from build123d import *

# Parameters (mm, degrees)
EXTRUDE_1_DEPTH     = 455
SKETCH_3_R          = 2.1
CUT_EXTRUDE_1_DEPTH = 466.453246739
SKETCH_7_W          = 87.07
SKETCH_7_H          = 105
CUT_EXTRUDE_2_DEPTH = 10


with BuildPart() as part:
    # 草图2 → 凸台-拉伸1 (new body)
    with BuildSketch(Plane.XY):
        Polygon((-98, -1), (-96.845299462, 1), (96.915299462, 1), (98.07, -1), align=None)
    extrude(amount=-EXTRUDE_1_DEPTH)

    # 草图3 → 切除-拉伸1 (cut, through all)
    with BuildSketch(Plane(origin=(0, -1, 0), x_dir=(-1, 0, 0), z_dir=(0, -1, 0))):
        with Locations(Location((78, 35, 0), (0, 0, 90))):
            Circle(SKETCH_3_R)
        with Locations(Location((78, 55, 0), (0, 0, 90))):
            Circle(SKETCH_3_R)
        with Locations(Location((-78, 55, 0), (0, 0, 270))):
            Circle(SKETCH_3_R)
        with Locations(Location((-78, 35, 0), (0, 0, 270))):
            Circle(SKETCH_3_R)
        with Locations(Location((-78, 420, 0), (0, 0, 90))):
            Circle(SKETCH_3_R)
        with Locations(Location((-78, 400, 0), (0, 0, 90))):
            Circle(SKETCH_3_R)
        with Locations(Location((78, 400, 0), (0, 0, 270))):
            Circle(SKETCH_3_R)
        with Locations(Location((78, 420, 0), (0, 0, 270))):
            Circle(SKETCH_3_R)
    extrude(amount=-CUT_EXTRUDE_1_DEPTH, mode=Mode.SUBTRACT)

    # 草图7 → 切除-拉伸2 (cut)
    with BuildSketch(Plane.XZ.offset(1)):
        with Locations((0.035, -302.5)):
            Rectangle(SKETCH_7_W, SKETCH_7_H)
    extrude(amount=-CUT_EXTRUDE_2_DEPTH, mode=Mode.SUBTRACT)


solid = part.part
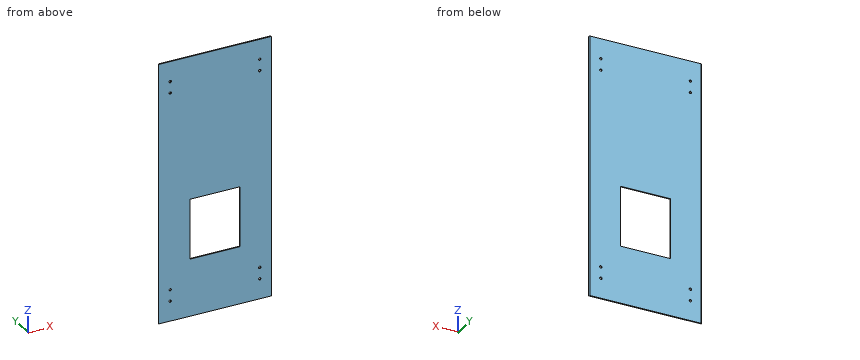
Input: part model. Units: mm. Frame: model coordinates. Give positions to 0.01 mm unless a question says otherwise; leave off trailing zeros. Write each loop counter-clockwise with the first axis right and the second up, starting at its lowest first coordinate (ties: lowest second). Pieces come first, ordered by that corner, then holes. Notation, with made-up numbers: M 46.5,78.25 L 72.5,78.25 A11 ccw 72.5,90.25 Z; hole C -13,76.25 d10. An arc over 180 degrees is marked long. Write item = value, one per line. Start each with the question number.
1) Cut plane B-B on z = -298.5. Return the cut outline in (x, y).
2) Material intervals for line 1 along X through (y, z) = (-0.5, -400); line 2 along Z through (x, y) = (-5.5, 0.65); line 3 along X through (y, z) = (0.8, -55), sorted ascending. Write a range as [from, to].
3) Cut plane C-C on y = -0.65. Count the separate pieces of the cut face and the enclosed holes in it, then the cut area to 3 significant figures.
4) First-contact query: pin 1 Ø1 at (y, z) = (0.5, -89) entering from +X; pin 2 Ø1 at (y, z) = (1, -235.5) entering from +X; pin 3 Ø4 at (x, z) = (-78, -55) entering from -Y; pin 4 Ø1 at (y, z) = (0.5, -351.5) entering from -X. Flat tips, straight axial feed; report the tip coordinate or a pass-through.
5) Cut plane A-A on x = -2. Return the cut outline in (y, z).
Solved:
q1.outline = M -98,-1 L -43.5,-1 L -43.5,1 L -96.85,1 Z; M 43.57,-1 L 98.07,-1 L 96.92,1 L 43.57,1 Z
q2.line_1 = [-97.71, -80.1], [-75.9, 75.9], [80.1, 97.78]
q2.line_2 = [-455, -355], [-250, 0]
q2.line_3 = [-96.96, -80.1], [-75.9, 75.9], [80.1, 97.03]
q3.separate_pieces = 1
q3.enclosed_holes = 9
q3.area = 79,800 mm2
q4.pin_1 = 97.49
q4.pin_2 = 97.2
q4.pin_3 = through
q4.pin_4 = -97.42
q5.outline = M -1,-455 L 1,-455 L 1,-355 L -1,-355 Z; M -1,-250 L 1,-250 L 1,0 L -1,0 Z
